Model file for the job. Use its own axes, mm. Face numbers are marked on the shaded views. A direction names the side the tool comes from. Coordinates: 2 decimals unless noted, no trailing zeros. Write each loop counter-clockwise with the first axis right and the second up, starting at its lowest first coordinate (ties: lowest second). Pieces come first, ordered by that corner, then holes. Notation, with made-up numbers: (19.25, -6) - (69.25, -6) arc R19 ccw to (69.25, 30) - close; hole circle Ø5 at (-32, 43). An arc over 180 degrees is marked (long way). Put each result on its own line as item: value. Start each with the question number.
1. Saw through at B-B, the plane z = 145. Write the cut outline in (x, y), plus the area to 3 significant figures.
2. Drop a flat-ended pin along its axis: P1, Ø8, axis at x = 80, z = 249.5, coming from the +Y side. Give the stop position or say it passes through.
3. Which spindle directions (+Z, -Z, +X, -X, +Y, -Y) get a long thin tool onto all of the face, cutting with end or side? Do the marked faces 4 and 5. Say none if no direction does.
4. Saw through at A-A, the plane y = -157.5. Write the cut outline in (x, z).
5. Saw through at C-C, the plane x = -158. Write the cut outline in (y, z), plus the area to 4 significant figures.
6. Pull direction X, two halves, no side cores. Call the marked faces 1, 2 and 3: released by +X, released by -X, zero draft, split by the parting line, or undercut.
7. Drill centre lines: L1, parallel to X at y = -129, z = 47.5; L2, parallel to Y at x = -161, z = 324.5. Where is each one in solid material? Low to high. Write a range as from..to.
```python
from build123d import *

# Parameters (mm, degrees)
SKETCH_1_W            = 420
SKETCH_1_H            = 480
EXTRUDE_1_DEPTH       = 5
FILLET_1_R            = 5
EXTRUDE_START         = 385
EXTRUDE_3_DEPTH       = 385
CUT_EXTRUDE_START     = -5
CUT_EXTRUDE_2_DEPTH   = 5
SHEET_START           = 5
SHEET_METAL_1_DEPTH   = 385
SHEET_METAL_1_2_DEPTH = 385


# Read off the part's stored shape, not the designer's step: 转换实体1
with BuildPart() as part:
    # Sketch 1 → 凸台-拉伸1 (new body)
    with BuildSketch(Plane.XY):
        Rectangle(SKETCH_1_W, SKETCH_1_H)
    extrude(amount=EXTRUDE_1_DEPTH)

    # 圆角1
    fillet_1_edges = [part.edges().sort_by_distance(p)[0] for p in [
        (210, -240, 2.5),
        (-210, -240, 2.5),
    ]]
    fillet(fillet_1_edges, radius=FILLET_1_R)

    # 草图4 → 凸台-拉伸3 (add)
    with BuildSketch(Plane.XY.offset(5).offset(EXTRUDE_START)):
        with BuildLine():
            Line((-205, 240), (-205, -235))
            Line((-205, -235), (205, -235))
            Line((205, -235), (205, 240))
            Line((205, 240), (210, 240))
            Line((210, 240), (210, -235))
            ThreePointArc((210, -235), (208.535533906, -238.535533906), (205, -240))
            Line((205, -240), (-205, -240))
            ThreePointArc((-205, -240), (-208.535533906, -238.535533906), (-210, -235))
            Line((-210, -235), (-210, 240))
            Line((-210, 240), (-205, 240))
        make_face()
    extrude(amount=-EXTRUDE_3_DEPTH)

    # 草图5 → 切除-拉伸2 (cut)
    with BuildSketch(Plane(origin=(0, 0, 0), x_dir=(-1, 0, 0), z_dir=(0, 0, -1)).offset(CUT_EXTRUDE_START)):
        with BuildLine():
            Line((-205, -240), (205, -240))
            ThreePointArc((205, -240), (208.535533906, -238.535533906), (210, -235))
            Line((210, -235), (210, 240))
            Line((210, 240), (-210, 240))
            Line((-210, 240), (-210, -235))
            ThreePointArc((-210, -235), (-208.535533906, -238.535533906), (-205, -240))
        make_face()
    extrude(amount=CUT_EXTRUDE_2_DEPTH, mode=Mode.SUBTRACT)

    # Sheet Metal 1 outline → Sheet Metal 1 (cut)
    with BuildSketch(Plane.XY.offset(SHEET_START)):
        with BuildLine():
            Line((-205, -240), (-200, -240))
            ThreePointArc((-200, -240), (-207.071067812, -237.071067812), (-210, -230))
            Line((-210, -230), (-210, -235))
            ThreePointArc((-210, -235), (-208.535533906, -238.535533906), (-205, -240))
        make_face()
        with BuildLine():
            ThreePointArc((210, -230), (207.071067812, -237.071067812), (200, -240))
            Line((200, -240), (205, -240))
            ThreePointArc((205, -240), (208.535533906, -238.535533906), (210, -235))
            Line((210, -235), (210, -230))
        make_face()
    extrude(amount=SHEET_METAL_1_DEPTH, mode=Mode.SUBTRACT)

    # Sheet Metal 1 2 outline → Sheet Metal 1 2 (add)
    with BuildSketch(Plane.XY.offset(SHEET_START)):
        with BuildLine():
            Line((-205, -235), (-200, -235))
            ThreePointArc((-200, -235), (-203.535533906, -233.535533906), (-205, -230))
            Line((-205, -230), (-205, -235))
        make_face()
        with BuildLine():
            ThreePointArc((205, -230), (203.535533906, -233.535533906), (200, -235))
            Line((200, -235), (205, -235))
            Line((205, -235), (205, -230))
        make_face()
    extrude(amount=SHEET_METAL_1_2_DEPTH)


solid = part.part
```
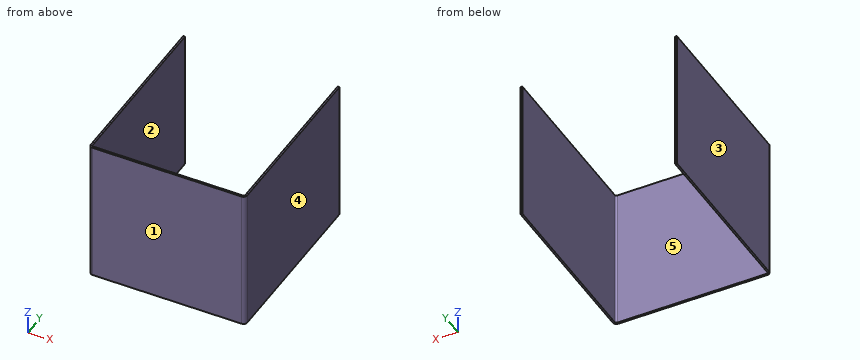
Final values:
1. outline: (-210, -230) arc R10 ccw to (-200, -240) - (200, -240) arc R10 ccw to (210, -230) - (210, 240) - (205, 240) - (205, -230) arc R5 cw to (200, -235) - (-200, -235) arc R5 cw to (-205, -230) - (-205, 240) - (-210, 240) - close
1. area: 6,820 mm²
2. P1: stops at y = -235
3. face 4: +Z, -Z, +X, +Y, -Y
3. face 5: +Z, -Z, +Y
4. outline: (-210, 5) - (-205, 5) - (-205, 390) - (-210, 390) - close; (205, 5) - (210, 5) - (210, 390) - (205, 390) - close
5. outline: (-240, 5) - (-235, 5) - (-235, 390) - (-240, 390) - close
5. area: 1,925 mm²
6. face 1: zero draft
6. face 2: undercut
6. face 3: released by -X
7. L1: x = -210..-205, 205..210
7. L2: y = -240..-235
